from build123d import *

# Parameters (mm, degrees)
F0_R          = 57.15
F1_DEPTH      = 12.7
F1_DEPTH_BACK = 12.7
F2_DEPTH      = 2.54
F2_DEPTH_BACK = 2.54
F4_T3_DEPTH   = 63.8207499086
F4_S4_R       = 7.62
F4_T5_DEPTH   = 35
F4_S6_R       = 44.45
F4_T7_DEPTH   = 35
F4_T10_DEPTH  = 63.0657347927
F4_S11_R      = 7.62
F4_T12_DEPTH  = 36
F4_S13_R      = 44.45
F4_T14_DEPTH  = 36
F4_T17_DEPTH  = 63.4473233417
F4_S18_R      = 7.62
F4_T19_DEPTH  = 34
F4_S20_R      = 44.45
F4_T21_DEPTH  = 34


# Not quite as in the source:
# - a fillet or chamfer that OpenCascade refuses, or shapes differently, is made with other operations: its cross-section is extruded or revolved along the edge and cut away or added


with BuildPart() as f1:
    # F0 (on Front) → F1 (new body, two sides)
    with BuildSketch(Plane.XZ) as f1_sk:
        Circle(F0_R)
        with BuildLine():
            ThreePointArc((30.2978338322, 32.5245102204), (40.7586875024, 17.7350470278), (44.45, 0))
            ThreePointArc((44.45, 0), (38.1514443262, -22.8094233996), (21.0407853398, -39.1546657793))
            ThreePointArc((21.0407853398, -39.1546657793), (8.0824234514, -43.7090028616), (-5.6476952972, -44.0897498046))
            ThreePointArc((-5.6476952972, -44.0897498046), (-30.9360762044, -31.9180464483), (-43.8918074796, -7.0222315665))
            ThreePointArc((-43.8918074796, -7.0222315665), (-44.0755738858, 5.7572811841), (-40.6153867658, 18.0608100003))
            ThreePointArc((-40.6153867658, 18.0608100003), (-21.1284803601, 39.1074138454), (7.15605679, 43.8701874992))
            ThreePointArc((7.15605679, 43.8701874992), (19.5673089339, 39.9114384743), (30.2978338322, 32.5245102204))
        make_face(mode=Mode.SUBTRACT)
    extrude(amount=F1_DEPTH)
    extrude(f1_sk.sketch, amount=-F1_DEPTH_BACK)



with BuildPart() as f1b:
    # F0 (on Front) → F1, piece 2 (new body, two sides)
    with BuildSketch(Plane.XZ) as f1_2_sk:
        with BuildLine():
            ThreePointArc((7.62, 0), (7.1992672661, 2.4969883522), (5.9835299656, 4.7182379285))
            ThreePointArc((5.9835299656, 4.7182379285), (3.3250133071, 6.8562880998), (0, 7.62))
            ThreePointArc((0, 7.62), (-2.66023415, 7.1405569998), (-4.9857096013, 5.7625601751))
            ThreePointArc((-4.9857096013, 5.7625601751), (-6.930205883, 3.168066669), (-7.62, 0))
            ThreePointArc((-7.62, 0), (-6.4667392377, -4.030593459), (-3.3560410415, -6.8411540348))
            ThreePointArc((-3.3560410415, -6.8411540348), (0.7135883563, -7.5865138013), (4.5728511754, -6.0953615256))
            ThreePointArc((4.5728511754, -6.0953615256), (6.815773102, -3.407291743), (7.62, 0))
        make_face()
    extrude(amount=F1_DEPTH)
    extrude(f1_2_sk.sketch, amount=-F1_DEPTH_BACK)


with BuildPart() as f1_1:
    add(f1.part)

    add(f1b.part)  # F2 merges F1b
    # F0 (on Front) → F2 (join, two sides)
    with BuildSketch(Plane.XZ) as f2_sk:
        with BuildLine():
            Line((5.9835299656, 4.7182379285), (30.2978338322, 32.5245102204))
            ThreePointArc((30.2978338322, 32.5245102204), (19.5673089339, 39.9114384743), (7.15605679, 43.8701874992))
            Line((7.15605679, 43.8701874992), (0, 7.62))
            ThreePointArc((0, 7.62), (3.3250133071, 6.8562880998), (5.9835299656, 4.7182379285))
        make_face()
        Polygon((21.6807832905, 31.4497899136), (4.4864523225, 12.7544701099), (10.4806591381, 37.4370446242), align=None, mode=Mode.SUBTRACT)
        with BuildLine():
            Line((-4.9857096013, 5.7625601751), (-40.6153867658, 18.0608100003))
            ThreePointArc((-40.6153867658, 18.0608100003), (-44.0755738858, 5.7572811841), (-43.8918074796, -7.0222315665))
            Line((-43.8918074796, -7.0222315665), (-7.62, 0))
            ThreePointArc((-7.62, 0), (-6.930205883, 3.168066669), (-4.9857096013, 5.7625601751))
        make_face()
        Polygon((-35.8506757944, 12.6760325764), (-11.6935795524, 4.8278034033), (-36.6305463748, 0), align=None, mode=Mode.SUBTRACT)
        with BuildLine():
            ThreePointArc((-5.6476952972, -44.0897498046), (8.0824234514, -43.7090028616), (21.0407853398, -39.1546657793))
            Line((21.0407853398, -39.1546657793), (4.5728511754, -6.0953615256))
            ThreePointArc((4.5728511754, -6.0953615256), (0.7135883563, -7.5865138013), (-3.3560410415, -6.8411540348))
            Line((-3.3560410415, -6.8411540348), (-5.6476952972, -44.0897498046))
        make_face()
        Polygon((-1.0400637192, -38.1721799109), (0.5196774415, -12.8201147581), (11.428419692, -35.7582782093), align=None, mode=Mode.SUBTRACT)
    extrude(amount=F2_DEPTH)
    extrude(f2_sk.sketch, amount=-F2_DEPTH_BACK)

    # F3: fillet of radius 7.62 on 2 edges, made by hand

    # F3_s1 → F3_t2 (revolve, cut)
    with BuildSketch(Plane(origin=(0, 0, 0), x_dir=(0, 1, 0), z_dir=(0.8977892434, 0, -0.4404253335))):
        with BuildLine():
            ThreePointArc((-5.08, -7.62), (-10.4681536726, -5.3881536726), (-12.7, 0))
            Line((-12.7, 0), (-12.7, -7.62))
            Line((-12.7, -7.62), (-5.08, -7.62))
        make_face()
    revolve(axis=Axis((0, -12.7, 0), (0, 1, 0)), mode=Mode.SUBTRACT)

    # F3_s3 → F3_t4 (revolve, cut)
    with BuildSketch(Plane(origin=(0, 0, 0), x_dir=(0, 1, 0), z_dir=(-0.8977892434, 0, 0.4404253335))):
        with BuildLine():
            ThreePointArc((5.08, 7.62), (10.4681536726, 5.3881536726), (12.7, 0))
            Line((12.7, 0), (12.7, 7.62))
            Line((12.7, 7.62), (5.08, 7.62))
        make_face()
    revolve(axis=Axis((0, 12.7, 0), (0, -1, 0)), mode=Mode.SUBTRACT)

    # F4: chamfer of 5.08 on 7 edges, made by hand


with BuildPart() as f4_tool1:
    # F4_s2 → F4_t3 (new body)
    with BuildSketch(Plane(origin=(6.116948919, 0, -2.1113793882), x_dir=(0, 1, 0), z_dir=(-0.9452735615, 0, 0.326278859))):
        Polygon((-2.54, 1.2595358599), (2.54, -3.8204641401), (-2.54, -3.8204641401), align=None)
    extrude(amount=F4_T3_DEPTH)

    # F4_s4 → F4_t5 (cut, symmetric)
    with BuildSketch(Plane.XZ):
        Circle(F4_S4_R)
    extrude(amount=F4_T5_DEPTH, both=True, mode=Mode.SUBTRACT)

    # F4_s6 → F4_t7 (intersect, symmetric)
    with BuildSketch(Plane.XZ):
        Circle(F4_S6_R)
    extrude(amount=F4_T7_DEPTH, both=True, mode=Mode.INTERSECT)


with BuildPart() as f4_tool8:
    # F4_s9 → F4_t10 (new body)
    with BuildSketch(Plane(origin=(-3.6688529254, 0, -4.1957657518), x_dir=(0, 1, 0), z_dir=(0.6582564125, 0, 0.7527937934))):
        Polygon((-2.54, 3.6814461509), (2.54, -1.3985538491), (-2.54, -1.3985538491), align=None)
    extrude(amount=F4_T10_DEPTH)

    # F4_s11 → F4_t12 (cut, symmetric)
    with BuildSketch(Plane.XZ):
        Circle(F4_S11_R)
    extrude(amount=F4_T12_DEPTH, both=True, mode=Mode.SUBTRACT)

    # F4_s13 → F4_t14 (intersect, symmetric)
    with BuildSketch(Plane.XZ):
        Circle(F4_S13_R)
    extrude(amount=F4_T14_DEPTH, both=True, mode=Mode.INTERSECT)


with BuildPart() as f4_tool15:
    # F4_s16 → F4_t17 (new body)
    with BuildSketch(Plane(origin=(0.3702740347, 0, 6.0184418339), x_dir=(0, 1, 0), z_dir=(-0.0614071323, 0, -0.9981128013))):
        Polygon((-2.54, 2.1503881258), (2.54, -2.9296118742), (-2.54, -2.9296118742), align=None)
    extrude(amount=F4_T17_DEPTH)

    # F4_s18 → F4_t19 (cut, symmetric)
    with BuildSketch(Plane.XZ):
        Circle(F4_S18_R)
    extrude(amount=F4_T19_DEPTH, both=True, mode=Mode.SUBTRACT)

    # F4_s20 → F4_t21 (intersect, symmetric)
    with BuildSketch(Plane.XZ):
        Circle(F4_S20_R)
    extrude(amount=F4_T21_DEPTH, both=True, mode=Mode.INTERSECT)


with BuildPart() as f4_tool22:
    # F4_s23 → F4_t24 (revolve)
    with BuildSketch(Plane(origin=(0, 0, 0), x_dir=(0, 1, 0), z_dir=(-0.8808698713, 0, -0.4733585003))):
        Polygon((-7.62, 44.45), (-12.7, 49.53), (-12.7, 44.45), align=None)
    revolve(axis=Axis((0, -12.7, 0), (0, -1, 0)))


with BuildPart() as f4_tool25:
    # F4_s26 → F4_t27 (revolve)
    with BuildSketch(Plane(origin=(0, 0, 0), x_dir=(0, 1, 0), z_dir=(0.8808698713, 0, 0.4733585003))):
        Polygon((7.62, -44.45), (12.7, -49.53), (12.7, -44.45), align=None)
    revolve(axis=Axis((0, 12.7, 0), (0, 1, 0)))


with BuildPart() as f4_tool28:
    # F4_s29 → F4_t30 (revolve)
    with BuildSketch(Plane.XY):
        Polygon((52.07, 12.7), (57.15, 7.62), (57.15, 12.7), align=None)
    revolve(axis=Axis((0, 12.7, 0), (0, -1, 0)))


with BuildPart() as f4_tool31:
    # F4_s32 → F4_t33 (revolve)
    with BuildSketch(Plane.XY):
        Polygon((52.07, -12.7), (57.15, -7.62), (57.15, -12.7), align=None)
    revolve(axis=Axis((0, -12.7, 0), (0, -1, 0)))


with BuildPart() as f1_2:
    add(f1_1.part)

    # F4_t34: cut F4_tool1, F4_tool8, F4_tool15, F4_tool22, F4_tool25, F4_tool28, F4_tool31
    add([f4_tool1.part, f4_tool8.part, f4_tool15.part, f4_tool22.part, f4_tool25.part, f4_tool28.part, f4_tool31.part], mode=Mode.SUBTRACT)


solid = f1_2.part
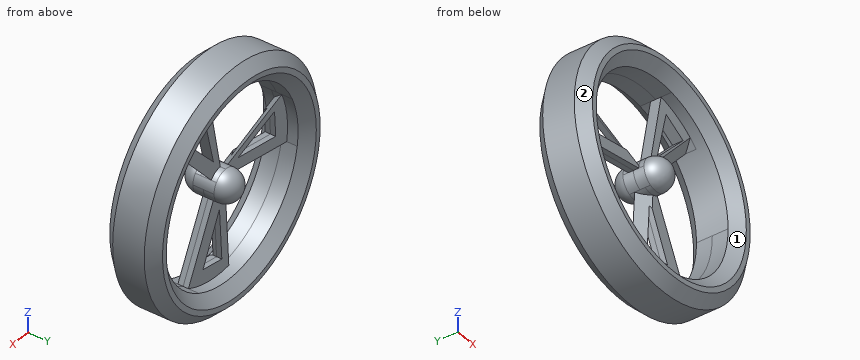
For this review, take the finished solid that the model builds, in its own axes (mm). Face numbers are marked on the shaded views. Give positions to 0.01 mm unless a question says otherwise; leave off trailing zeros. Answer as a JSON object with one key per item and string values. Group by question number.
Q1. For probe 1 along X at (y, z) = (2.5, 19); probe 2 along Z at (x, y) = (6.5, -5.5); probe 3 along Z at (x, y) = (-18, -2), list the stretches that pass through material, from the lowest coordinate up. Write a range as [from, to].
Q2. Mouldability with a two-part tool opening along X and no side actions: class the marked faces 1 and 2 as +X half, -X half, draft (parallel to the pull), parting line (faces both ways), or undercut.
Q3. Add section A-A on z = -10.5. Give the number of separate pieces and of enclosed holes in the cut face, and give its area (3 significant figures).
Q4. Insertion check: P1, Ø1, axis at x = 41.5, z = 15.5, coming from the +Y side; P2, Ø10, axis at y = 0, z = -43.5, coming from the -X side; P3, Ø1, axis at y = -8, z = -7.5, coming from the +X side. Each pin has a flat end and moves straight along its axis. Give the tip position at first contact, or say it passes through.
Checked values:
{
 "1": {"probe 1": "[-53.9, -40.18], [2.25, 6], [10.23, 18.42], [40.18, 53.9]", "probe 2": "[-56.78, -43.97], [-3.95, 3.95], [43.97, 56.78]", "probe 3": "[-54.24, -40.64], [-2.01, 3.61], [40.64, 54.24]"},
 "2": {"face 1": "undercut", "face 2": "parting line"},
 "3": {"separate pieces": "3", "enclosed holes": "0", "area": "594 mm²"},
 "4": {"P1": "y = 7.97", "P2": "x = -42.24", "P3": "x = 56.7"}
}
